from build123d import *

# Parameters (mm, degrees)
F0_W     = 6.6
F0_H     = 6.6
F0_R     = 3.15
F1_DEPTH = 1.5
F2_DEPTH = 3.1
F3_DEPTH = 3.101
F4_DEPTH = 1.5


with BuildPart() as f1:
    # F0 (on Top) → F1 (new body)
    with BuildSketch(Plane.XY):
        with BuildLine():
            Line((3.5, 5.5), (-3.5, 5.5))
            ThreePointArc((-3.5, 5.5), (-4.914214, 4.914214), (-5.5, 3.5))
            Line((-5.5, 3.5), (-5.5, -3.5))
            ThreePointArc((-5.5, -3.5), (-4.914214, -4.914214), (-3.5, -5.5))
            Line((-3.5, -5.5), (3.5, -5.5))
            ThreePointArc((3.5, -5.5), (4.914214, -4.914214), (5.5, -3.5))
            Line((5.5, -3.5), (5.5, 3.5))
            ThreePointArc((5.5, 3.5), (4.914214, 4.914214), (3.5, 5.5))
        make_face()
        with BuildLine():
            ThreePointArc((-4, 2.5), (-3.56066, 3.56066), (-2.5, 4))
            Line((-2.5, 4), (2.5, 4))
            ThreePointArc((2.5, 4), (3.56066, 3.56066), (4, 2.5))
            Line((4, 2.5), (4, -2.5))
            ThreePointArc((4, -2.5), (3.56066, -3.56066), (2.5, -4))
            Line((2.5, -4), (-2.5, -4))
            ThreePointArc((-2.5, -4), (-3.56066, -3.56066), (-4, -2.5))
            Line((-4, -2.5), (-4, 2.5))
        make_face(mode=Mode.SUBTRACT)
        with BuildLine():
            Line((2.5, 4), (-2.5, 4))
            ThreePointArc((-2.5, 4), (-3.56066, 3.56066), (-4, 2.5))
            Line((-4, 2.5), (-4, -2.5))
            ThreePointArc((-4, -2.5), (-3.56066, -3.56066), (-2.5, -4))
            Line((-2.5, -4), (2.5, -4))
            ThreePointArc((2.5, -4), (3.56066, -3.56066), (4, -2.5))
            Line((4, -2.5), (4, 2.5))
            ThreePointArc((4, 2.5), (3.56066, 3.56066), (2.5, 4))
        make_face()
        Rectangle(F0_W, F0_H, mode=Mode.SUBTRACT)
        Rectangle(F0_W, F0_H)
        Circle(F0_R, mode=Mode.SUBTRACT)
        Circle(F0_R)
    extrude(amount=F1_DEPTH)

    # F0 (on Top) → F2 (join)
    with BuildSketch(Plane.XY):
        with BuildLine():
            Line((2.5, 4), (-2.5, 4))
            ThreePointArc((-2.5, 4), (-3.56066, 3.56066), (-4, 2.5))
            Line((-4, 2.5), (-4, -2.5))
            ThreePointArc((-4, -2.5), (-3.56066, -3.56066), (-2.5, -4))
            Line((-2.5, -4), (2.5, -4))
            ThreePointArc((2.5, -4), (3.56066, -3.56066), (4, -2.5))
            Line((4, -2.5), (4, 2.5))
            ThreePointArc((4, 2.5), (3.56066, 3.56066), (2.5, 4))
        make_face()
        Rectangle(F0_W, F0_H, mode=Mode.SUBTRACT)
        Rectangle(F0_W, F0_H)
        Circle(F0_R, mode=Mode.SUBTRACT)
        Circle(F0_R)
    extrude(amount=F2_DEPTH)

    # F0 (on Top) → F3 (cut, through all)
    with BuildSketch(Plane.XY):
        Circle(F0_R)
    extrude(amount=F3_DEPTH, mode=Mode.SUBTRACT)

    # F0 (on Top) → F4 (cut)
    with BuildSketch(Plane.XY):
        Rectangle(F0_W, F0_H)
        Circle(F0_R, mode=Mode.SUBTRACT)
        Circle(F0_R)
    extrude(amount=F4_DEPTH, mode=Mode.SUBTRACT)


solid = f1.part
The listing builds one solid part. Answer for the finished solid, in the listing's coordinates (mm). A direction names the side the tool comes from. Coordinates: 2 decimals unless noted, no trailing zeros. Loops run counter-clockwise (first coordinate to the right, second up) from the corner with the lowest first, then second, coordinate; pieces in that order, holes last. Notation, with made-up numbers: (-11, 19.25) -> (43, 19.25) arc R21 cw to (43, 29.25) -> close; hole circle Ø1 at (17, 75). An arc over 180 degrees is marked (long way). Write item = value, one per line. Start each with the question number.
1) A tool of negligible diameter and unlimited length cuts with its end or side. For faces 4 (the face through (0, -3.3, 1)), 5 (the face through (-3.55, 3.57, 2.29)), 6 (the face through (3.57, 3.55, 2.29)), 7 (the face through (5, 0, 1.5)), from which of +Z, -Z, +X, -X, +Y, -Y can it reach the whole face along a straight path? Write none if from no direction.
2) A cutting plane is placed at A-A (y = 0). Give the vertices of the cut face in (x, z).
3) A cutting plane is placed at C-C (z = 2.2). Give the vertices of the cut face in (x, y), then the cut area to 3 significant figures.
4) Given pin 1 Ø1.3 at (y, z) = (1, 2.5) entering from -X; pin 2 Ø5 at (x, y) = (0, 0) entering from +Z; pin 3 Ø1.8 at (x, z) = (0.5, 2.5) entering from -Y; pin 4 Ø1.3 at (y, z) = (0, 2.5) entering from +X, each flat-ended and moving along its own axis, determine where each tip first touches the part or whether it passes through.
5) The mould has two halves that part along X. Classify faces 1 (the face through (-5.5, 0, 1)), 2 (the face through (0, -4, 2)), 3 (the face through (3.3, 0, 1)): released by +X, released by -X, zero draft, split by the parting line, or undercut.
6) Straight lines are drawn through the part: line 1 (X direction, y = -3, z = 1.35); line 2 (Y direction, x = 0, z = 2.55). For each, find the intervals that lie inside material, in ascending order. Write a range as from..to.
Responses:
q1.face_4 = -Z
q1.face_5 = +Z, -X, +Y
q1.face_6 = +Z, +X, +Y
q1.face_7 = +Z
q2.outline = (-5.5, 0) -> (-3.3, 0) -> (-3.3, 1.5) -> (-3.15, 1.5) -> (-3.15, 3.1) -> (-4, 3.1) -> (-4, 1.5) -> (-5.5, 1.5) -> close; (3.15, 1.5) -> (3.3, 1.5) -> (3.3, 0) -> (5.5, 0) -> (5.5, 1.5) -> (4, 1.5) -> (4, 3.1) -> (3.15, 3.1) -> close
q3.outline = (-4, -2.5) arc R1.5 ccw to (-2.5, -4) -> (2.5, -4) arc R1.5 ccw to (4, -2.5) -> (4, 2.5) arc R1.5 ccw to (2.5, 4) -> (-2.5, 4) arc R1.5 ccw to (-4, 2.5) -> close; hole circle Ø6.3 at (0, 0)
q3.area = 30.9 mm²
q4.pin_1 = -4
q4.pin_2 = through
q4.pin_3 = -4
q4.pin_4 = 4
q5.face_1 = released by -X
q5.face_2 = zero draft
q5.face_3 = undercut
q6.line_1 = -5.5..-3.3, 3.3..5.5
q6.line_2 = -4..-3.15, 3.15..4
